Can you work these out from the model? Positions are in its coordinate system, mm. A direction names the side the tool comes from. Coordinates: 2 decimals unless noted, no trailing zeros. Order: outer loops, then holes, each group sorted by start corner. A loop starts at its lowest first (then second) coordinate and runs counter-clockwise, first axis right, second up. Notation, with made-up numbers: (-33, -36) -> (17, -36) arc R21 ccw to (17, -23) -> close; hole circle Ø2 at (70.5, -40). An arc over 180 degrees is marked (long way). Return JSON: item names as keys, results as strings. Group by question number.
1) If we section it at B-B, the plane z = 4: Please give me the cut outline in (x, y), then the cut area to 3 significant figures.
2) If I drill on probe 1 along X at (y, z) = (10, 18.25); probe 2 along X at (y, z) = (10.5, -3.5); probe 3 along Y at (x, z) = (23, 5.5), over which ranges is the centre line in solid material (lowest first)? Write a range as from..to.
3) For faces 1 (the cylindrical face through (20.38, 10.83, 5.37)), 2 (the flat face through (17, 10, -16)), 3 (the flat face through (-20, 10, -11)), which set-ups out of +Z, -Z, +X, -X, +Y, -Y let a thin tool reach every point of the face, with its end or its side?
4) If we section it at C-C, the plane y = 18: Please give me the cut outline in (x, z), then the cut area to 3 significant figures.
5) Thinking about a two-plate mould opening in Z: for faces 4 (the cylindrical face through (-23.596, 16.041, -0.815)), 5 (the flat face through (20, 10, -11)), 6 (the cylindrical face through (25.747, 10.121, -8.136)), which applies, +Z half, -Z half, draft (parallel to the pull), parting line (faces both ways), or undercut?
6) For pin 1 (8 mm diameter, centred on x = -12, z = -15.5, fed in from -Y); pin 2 (3 mm diameter, centred on y = 12, z = -14.5, fed in from -X); pin 3 (3 mm diameter, centred on y = 10, z = -14, fed in from +X); pin 4 (3 mm diameter, centred on x = 22.5, y = 8, fed in from -Z), each with a flat end and sliding along its axis, tell me the tip position at first contact or that it passes through.
7) If we section it at A-A, the plane x = 23: Please give me the cut outline in (y, z).
8) If we section it at D-D, the plane z = -2: Please give me the cut outline in (x, y), then the cut area to 3 significant figures.
from build123d import *

# Parameters (mm, degrees)
SKETCH1_R           = 5
SKETCH1_R_2         = 2.75
BOSS_EXTRUDE1_DEPTH = 20
SKETCH2_R           = 2.75
CUT_EXTRUDE1_DEPTH  = 33.5
SKETCH3_W           = 6.5
SKETCH3_H           = 32
CUT_EXTRUDE2_DEPTH  = 21


with BuildPart() as part:
    # Sketch1 → Boss-Extrude1 (new body)
    with BuildSketch(Plane(origin=(0, 0, 0), x_dir=(1, 0, 0), z_dir=(0, 1, 0))):
        Polygon((30, -21.5), (-30, -21.5), (-30, 11), (-17, 11), (-17, 21.5), (17, 21.5), (17, 11), (30, 11), align=None)
        with Locations((0, 3.5)):
            Circle(SKETCH1_R, mode=Mode.SUBTRACT)
        with Locations((-23, 3.5)):
            Circle(SKETCH1_R_2, mode=Mode.SUBTRACT)
        with Locations((-23, -14.5)):
            Circle(SKETCH1_R_2, mode=Mode.SUBTRACT)
        with Locations((23, 3.5)):
            Circle(SKETCH1_R_2, mode=Mode.SUBTRACT)
        with Locations((23, -14.5)):
            Circle(SKETCH1_R_2, mode=Mode.SUBTRACT)
    extrude(amount=BOSS_EXTRUDE1_DEPTH)

    # Sketch2 → Cut-Extrude1 (cut, through all)
    with BuildSketch(Plane(origin=(0, 0, -11), x_dir=(-1, 0, 0), z_dir=(0, 0, -1))):
        with Locations((-23, 10)):
            Circle(SKETCH2_R)
        with Locations((23, 10)):
            Circle(SKETCH2_R)
    extrude(amount=-CUT_EXTRUDE1_DEPTH, mode=Mode.SUBTRACT)

    # Sketch3 → Cut-Extrude2 (cut, through all)
    with BuildSketch(Plane.XZ):
        with Locations((30, -11)):
            Rectangle(SKETCH3_W, SKETCH3_H)
        with Locations((-30, -11)):
            Rectangle(SKETCH3_W, SKETCH3_H)
    extrude(amount=-CUT_EXTRUDE2_DEPTH, mode=Mode.SUBTRACT)


solid = part.part
Result sheet:
{
 "1": {"outline": "(-26.75, 0) -> (26.75, 0) -> (26.75, 20) -> (-26.75, 20) -> close; hole circle Ø5.5 at (-23, 10); hole circle Ø5.5 at (23, 10)", "area": "1,020 mm2"},
 "2": {"probe 1": "x = -30..-25.75, -20.25..20.25, 25.75..30", "probe 2": "x = -26.75..-25.75, -20.25..-5, 5..20.25, 25.75..26.75", "probe 3": "y = 0..7.25, 12.75..20"},
 "3": {"face 1": "+Z, -Z", "face 2": "-Z, +X, +Y, -Y", "face 3": "-Z, -X, +Y, -Y"},
 "4": {"outline": "(-30, 5) -> (-26.75, 5) -> (-26.75, -11) -> (-17, -11) -> (-17, -21.5) -> (17, -21.5) -> (17, -11) -> (26.75, -11) -> (26.75, 5) -> (30, 5) -> (30, 21.5) -> (-30, 21.5) -> close; hole circle Ø5.5 at (-23, -3.5); hole circle Ø5.5 at (-23, 14.5); hole circle Ø10 at (0, -3.5); hole circle Ø5.5 at (23, -3.5); hole circle Ø5.5 at (23, 14.5)", "area": "2,030 mm2"},
 "5": {"face 4": "undercut", "face 5": "-Z half", "face 6": "draft"},
 "6": {"pin 1": "stops at y = 0", "pin 2": "stops at x = -17", "pin 3": "stops at x = 17", "pin 4": "stops at z = -11"},
 "7": {"outline": "(0, -11) -> (7.25, -11) -> (7.25, -6.25) -> (0, -6.25) -> close; (0, -0.75) -> (7.25, -0.75) -> (7.25, 11.75) -> (0, 11.75) -> close; (0, 17.25) -> (7.25, 17.25) -> (7.25, 21.5) -> (0, 21.5) -> close; (12.75, -11) -> (20, -11) -> (20, -6.25) -> (12.75, -6.25) -> close; (12.75, -0.75) -> (20, -0.75) -> (20, 11.75) -> (12.75, 11.75) -> close; (12.75, 17.25) -> (20, 17.25) -> (20, 21.5) -> (12.75, 21.5) -> close"},
 "8": {"outline": "(-26.75, 0) -> (-25.3, 0) -> (-25.3, 8.5) arc R2.75 cw to (-25.3, 11.5) -> (-25.3, 20) -> (-26.75, 20) -> close; (-20.7, 0) -> (-4.77, 0) -> (-4.77, 20) -> (-20.7, 20) -> (-20.7, 11.5) arc R2.75 cw to (-20.7, 8.5) -> close; (4.77, 0) -> (20.7, 0) -> (20.7, 8.5) arc R2.75 cw to (20.7, 11.5) -> (20.7, 20) -> (4.77, 20) -> close; (25.3, 0) -> (26.75, 0) -> (26.75, 20) -> (25.3, 20) -> (25.3, 11.5) arc R2.75 cw to (25.3, 8.5) -> close", "area": "691 mm2"}
}
